```python
from build123d import *

# Parameters (mm, degrees)
CUT_EXTRUDE_1_DEPTH      = 39.448016854
CUT_EXTRUDE_1_DEPTH_BACK = 39.448016854
SKETCH_2_R               = 1.6


with BuildPart() as part:
    # 草图1 → 旋转1 (revolve)
    with BuildSketch(Plane.XY, mode=Mode.PRIVATE) as revolve_1_sk:
        Polygon((0, 0), (6, 0), (6, 2.5), (4, 2.5), (4, 36.5), (3.422649731, 37.5), (0, 37.5), align=None)
    revolve(revolve_1_sk.sketch.rotate(Axis((0, 0, 0), (0, -1, 0)), 90), axis=Axis((0, 0, 0), (0, -1, 0)))

    # 草图2 → 切除-拉伸1 (cut, two sides: drawn at the far end of the back side and taken through both)
    with BuildSketch(Plane.XY.offset(-CUT_EXTRUDE_1_DEPTH_BACK)):
        with Locations((0, 34)):
            Circle(SKETCH_2_R)
    extrude(amount=CUT_EXTRUDE_1_DEPTH + CUT_EXTRUDE_1_DEPTH_BACK, mode=Mode.SUBTRACT)


solid = part.part
```
Check sheet for the modelled part. Datum: model origin and axes. Units: mm. A direction names the side the tool comes from. Coordinates: 2 decimals unless noted, no trailing zeros. Write each loop counter-clockwise with the first axis right and the second up, starting at its lowest first coordinate (ties: lowest second). Pieces come first, ordered by that corner, then holes. Notation, with made-up numbers: (-18.5, 54.25) -> (0.5, 54.25) arc R27 cw to (0.5, 89.25) -> close; hole circle Ø10 at (7.25, -15). An arc over 180 degrees is marked (long way). Use a Markdown table: item, result.
1. Sectioned sample at A-A (z = 0). Enter the section's corners in (x, y), plus the area to 3 significant figures.
Reported:
| item | result |
|---|---|
| outline | (-6, 0) -> (6, 0) -> (6, 2.5) -> (4, 2.5) -> (4, 36.5) -> (3.42, 37.5) -> (-3.42, 37.5) -> (-4, 36.5) -> (-4, 2.5) -> (-6, 2.5) -> close; hole circle Ø3.2 at (0, 34) |
| area | 301 mm2 |
2. Go/stop test with flat-tipped pins: pin 1 Ø4 at (x, y) = (0, 34) entering from -Z; pin 2 Ø2 at (x, y) = (4, 5) entering from -Z; pin 3 Ø4 at (y, z) = (11.5, 4) entering from +X. Record where each tip stops, or that it passes through.
Reported:
| item | result |
|---|---|
| pin 1 | stops at z = -4 |
| pin 2 | stops at z = -2.65 |
| pin 3 | stops at x = 3.46 |
3. Sectioned sample at C-C (y = 13.5). Enter the section's corners in (x, z), plus the area to 3 significant figures.
Reported:
| item | result |
|---|---|
| outline | circle Ø8 at (0, 0) |
| area | 50.3 mm2 |
4. Scan lines: line 1 along Y through (x, z) = (0, -0.25); line 2 along X through (y, z) = (34, 1); line 3 along Y through (x, z) = (4.75, 0.25). Record each from-to range of solid material in increasing order.
Reported:
| item | result |
|---|---|
| line 1 | y = 0 to 32.4, 35.6 to 37.5 |
| line 2 | x = -3.87 to -1.6, 1.6 to 3.87 |
| line 3 | y = 0 to 2.5 |
5. Sectioned sample at D-D (y = 34). Enter the section's corners in (x, z), plus the area to 3 significant figures.
Reported:
| item | result |
|---|---|
| outline | (-1.6, -3.67) -> (-1.6, 3.67) arc R4 ccw to start; (1.6, -3.67) arc R4 ccw to (1.6, 3.67) -> close |
| area | 25.4 mm2 |
6. Release check for a two-part mould opening along Y. For faces 1 (the flat face through (3.92, 2.5, -1.42)), 2 (the flat face through (0, 0, 0)), 3 (the cylindrical face through (-1.802, 1.268, 5.723)), 4 (the cylindrical face through (0.74, 32.58, -0.06)) record: pulls with the +Y half, pulls with the -Y half, needs draft (parallel to the pull), parting line crosses it, or undercut.
Reported:
| item | result |
|---|---|
| face 1 | pulls with the +Y half |
| face 2 | pulls with the -Y half |
| face 3 | needs draft |
| face 4 | undercut |
7. Sectioned sample at B-B (x = 0). Enter the section's corners in (y, z).
Reported:
| item | result |
|---|---|
| outline | (0, -6) -> (2.5, -6) -> (2.5, -4) -> (32.4, -4) -> (32.4, 4) -> (2.5, 4) -> (2.5, 6) -> (0, 6) -> close; (35.6, -4) -> (36.5, -4) -> (37.5, -3.42) -> (37.5, 3.42) -> (36.5, 4) -> (35.6, 4) -> close |
8. Tool access check on faces 5 (the cylindrical face through (3.549, 19.738, 1.846)), 6 (the flat face through (0, 37.5, 0)). Record the directions out of +Z, -Z, +X, -X, +Y, -Y that give a thin tool (end or side, any length) a straight path to the whole face; none if there is none.
Reported:
| item | result |
|---|---|
| face 5 | +Y |
| face 6 | +Z, -Z, +X, -X, +Y |
